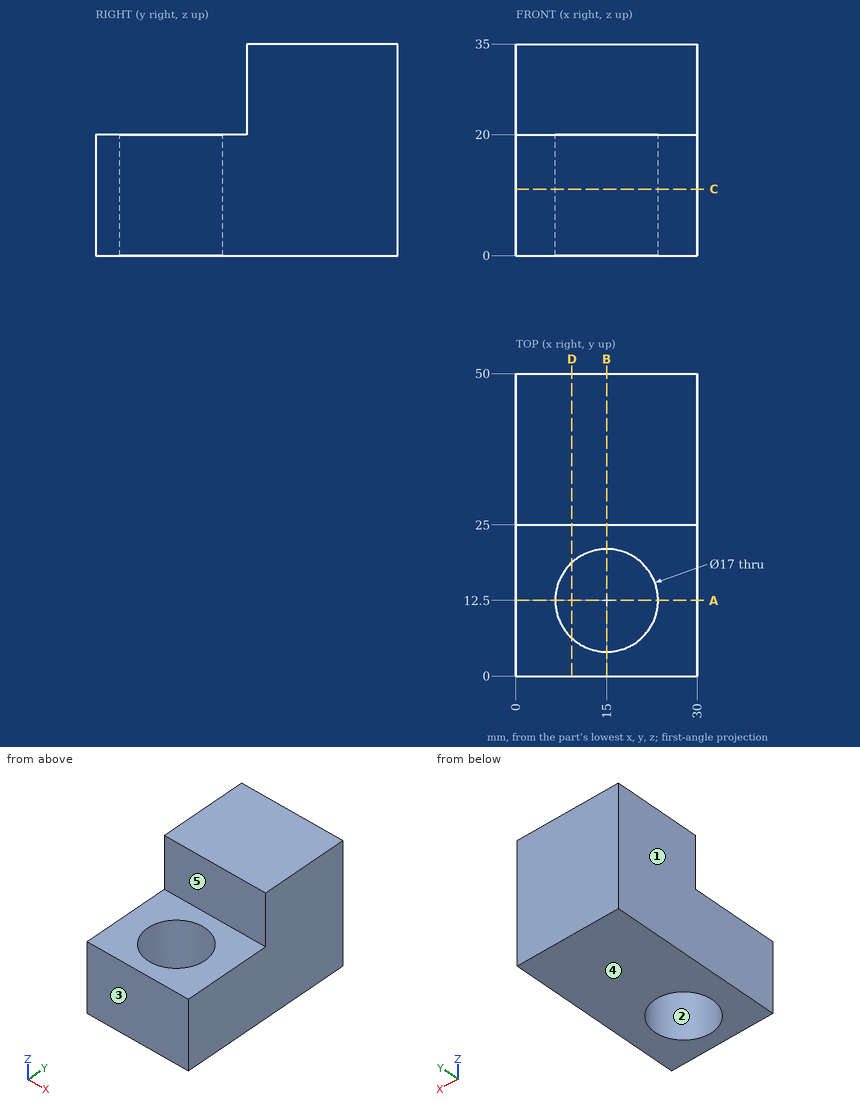
Could you check a few things on this drawing? It's one solid part, dimensions in mm from its lowest x, y, z. A direction names the side the tool comes from. Give positions to 0.01 mm unless a question says otherwise; leave off trailing zeros. Order: outer loops, then holes, each group sorted by start corner. A loop starts at its lowest first (then second) coordinate and runs counter-clockwise, first axis right, second up. Notation, with made-up numbers: (5.25, -11.75) -> (55.25, -11.75) arc R21 ccw to (55.25, -2.75) -> close; hole circle Ø9 at (69, 40.5). An arc over 180 degrees is marked (long way). Answer in a Markdown table with one row per item. Add a question column.
Item 1: Imagine slicing it at B-B (x = 15). List the corners of the cut face in (y, z) for me.
Item 2: I'm going to push flat-ended pins straight in: P1, Ø1.5, axis at x = 10, y = 16, coming from the -Z side; P2, Ø3, axis at x = 3.5, y = 9.5, coming from the +Z side; P3, Ø7.5, axis at x = 22.5, z = 28.5, coming from the -Y side. Where does each tip first touch, or does it pass through?
Item 3: Imagine slicing it at D-D (x = 9.25). List the corners of the cut face in (y, z) for me.
Item 4: Imagine slicing it at A-A (y = 12.5). List the corners of the cut face in (x, z) for me, and give its area (3 significant figures).
Item 5: Please list where these lines run through material, in increasing order: probe 1 along Y at (x, z) = (15, 8); probe 2 along Z at (x, y) = (23.5, 3); probe 3 along Y at (x, z) = (7, 28).
Item 6: We'd pull the mould along X, two halves only. Please class the marked faces 1, 2 and 3: pulls with the +X half, pulls with the -X half, needs draft (parallel to the pull), parting line crosses it, or undercut.
Item 7: Imagine slicing it at C-C (z = 11). List the corners of the cut face in (x, y) for me, and give its area (3 significant figures).
Item 8: For the marked faces 4 and 5, which set-ups out of +Z, -Z, +X, -X, +Y, -Y let a thin tool reach every point of the face, with its end or its side?
Result:
| question | item | result |
|---|---|---|
| 1 | outline | (0, 0) -> (4, 0) -> (4, 20) -> (0, 20) -> close; (21, 0) -> (50, 0) -> (50, 35) -> (25, 35) -> (25, 20) -> (21, 20) -> close |
| 2 | P1 | through |
| 2 | P2 | z = 20 |
| 2 | P3 | y = 25 |
| 3 | outline | (0, 0) -> (6.24, 0) -> (6.24, 20) -> (0, 20) -> close; (18.76, 0) -> (50, 0) -> (50, 35) -> (25, 35) -> (25, 20) -> (18.76, 20) -> close |
| 4 | outline | (0, 0) -> (6.5, 0) -> (6.5, 20) -> (0, 20) -> close; (23.5, 0) -> (30, 0) -> (30, 20) -> (23.5, 20) -> close |
| 4 | area | 260 mm2 |
| 5 | probe 1 | 0 to 4, 21 to 50 |
| 5 | probe 2 | 0 to 20 |
| 5 | probe 3 | 25 to 50 |
| 6 | face 1 | pulls with the -X half |
| 6 | face 2 | undercut |
| 6 | face 3 | needs draft |
| 7 | outline | (0, 0) -> (30, 0) -> (30, 50) -> (0, 50) -> close; hole circle Ø17 at (15, 12.5) |
| 7 | area | 1,270 mm2 |
| 8 | face 4 | -Z, +X, -X, +Y, -Y |
| 8 | face 5 | +Z, +X, -X, -Y |
